Input: part model. Units: mm. Frame: model coordinates. Round coordinates to 2 decimals unless told otherwise and drop trailing zeros. Loops run counter-clockwise (first coordinate to the right, second up) from the corner with the lowest first, then second, coordinate; pieces in that order, holes last. Notation, with made-up numbers: M 11,75 L 34,75 A21 cw 34,102 Z; hole C -16.75,35.5 d4. An arc over 180 degrees is marked long. Return JSON: item names as keys, results as strings. Group by question number.
1) Material intervals for line 1 (Z direction, x = -3, y = -10.75); line 2 (X direction, y = -14.5, z = -14.5); line 3 (X direction, y = -4.5, z = -8.5), sorted ascending. Write a range as from..to.
2) Section B-B (y = -5.25). Output: boundary loops of the cut face in (x, z).
3) Section C-C (z = -14). Output: boundary loops of the cut face in (x, y), plus the area to 3 significant figures.
4) Contact query for flat-ended pins moving along their axis: P1, Ø5.5, axis at y = -8, z = 31, coming from the -X side; P2, Ø10, axis at y = -11.5, z = -26.5, coming from the +X side; P3, Ø9, axis at x = -33, y = -6, coming from the -Z side. Output: stop coordinate, or through.
5) Section A-A (x = 15). Output: boundary loops of the cut face in (y, z), plus the area to 3 significant figures.
6) Section D-D (x = 71.5). Output: boundary loops of the cut face in (y, z), plus the area to 3 significant figures.
from build123d import *

# Parameters (mm, degrees)
F0_R     = 200
F1_DEPTH = 18


with BuildPart() as f1:
    # F0 (on Front) → F1 (new body)
    with BuildSketch(Plane.XZ):
        with Locations((-0.282222, -1.128889)):
            Circle(F0_R)
        Polygon((9, -9), (9, -45), (-9, -45), (-9, -9), (-45, -9), (-45, 9), (-9, 9), (-9, 45), (9, 45), (9, 9), (45, 9), (45, -9), align=None, mode=Mode.SUBTRACT)
    extrude(amount=F1_DEPTH)


solid = f1.part
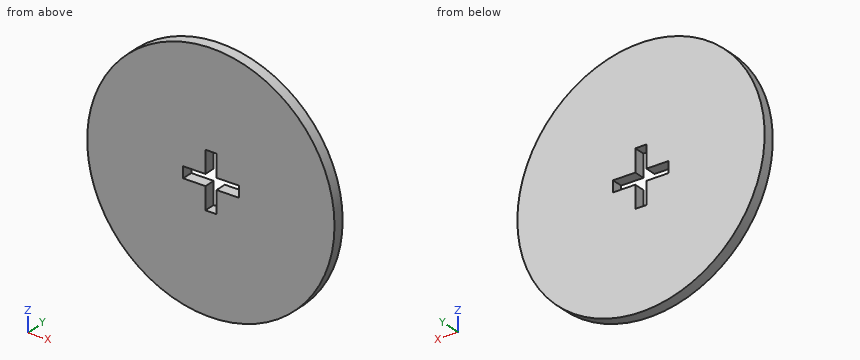
Returned:
{
 "1": {"line 1": "z = -201.11..-45, 45..198.85", "line 2": "x = -199.83..-9, 9..199.27", "line 3": "x = -200.15..-45, 45..199.58"},
 "2": {"outline": "C -0.28,-1.13 d400; hole M -45,-9 L -9,-9 L -9,-45 L 9,-45 L 9,-9 L 45,-9 L 45,9 L 9,9 L 9,45 L -9,45 L -9,9 L -45,9 Z"},
 "3": {"outline": "M -199.87,-18 L -9,-18 L -9,0 L -199.87,0 Z; M 9,-18 L 199.3,-18 L 199.3,0 L 9,0 Z", "area": "6,860 mm^2"},
 "4": {"P1": "stops at x = -198.11", "P2": "stops at x = 198.68", "P3": "stops at z = -199.13"},
 "5": {"outline": "M -18,-200.54 L 0,-200.54 L 0,-9 L -18,-9 Z; M -18,9 L 0,9 L 0,198.29 L -18,198.29 Z", "area": "6,850 mm^2"},
 "6": {"outline": "M -18,-187.8 L 0,-187.8 L 0,185.55 L -18,185.55 Z", "area": "6,720 mm^2"}
}
